Geometry check sheet. Reference: the model listing, model coordinates, mm. A direction names the side the tool comes from. Coordinates: 2 decimals unless noted, no trailing zeros. Write each loop counter-clockwise with the first axis right and the second up, starting at its lowest first coordinate (ties: lowest second). Pieces come first, ordered by that corner, then holes. Notation, with made-up numbers: (39, -12) -> (81, -12) arc R23 ccw to (81, 12) -> close; hole circle Ø4 at (10, 69.25). An arc over 180 degrees is marked (long way). One line per question, with ' | ' between items.
from build123d import *

# Parameters (mm, degrees)
F1_DEPTH = 25


with BuildPart() as f1:
    # F0 (on Right) → F1 (new body)
    with BuildSketch(Plane.YZ):
        with BuildLine():
            ThreePointArc((-42.22845, 60.540393), (-37.159315, 143.848694), (-61.121118, 223.797434))
            Line((-61.121118, 223.797434), (-85.621118, 223.797434))
            Line((-85.621118, 223.797434), (-85.621118, 299.997434))
            Line((-85.621118, 299.997434), (-110.621118, 299.997434))
            Line((-110.621118, 299.997434), (-110.621118, 224.997434))
            ThreePointArc((-110.621118, 224.997434), (-79.816037, 145.650842), (-78.79324, 60.540393))
            ThreePointArc((-78.79324, 60.540393), (-76.894776, -39.398884), (-38.776239, -131.802566))
            Line((-38.776239, -131.802566), (-16.268492, -131.802566))
            ThreePointArc((-16.268492, -131.802566), (-47.291443, -38.066293), (-42.22845, 60.540393))
        make_face()
    extrude(amount=F1_DEPTH)


solid = f1.part
1. Mould release check, pull along Z, two halves, no side actions. Record for faces 3 (the face through (12.325, -47.102, -39.444)), 4 (the face through (12, -28, -131.803)), 5 (the face through (12.325, -77.178, -38.02)), 6 (the face through (25, -67, 85)): released by +Z, released by -Z, zero draft, split by the parting line, or undercut.
Worked answers:
face 3: undercut | face 4: released by -Z | face 5: undercut | face 6: zero draft
2. Cross-section at A-A on x = 17. Record the boundary of the cut face in (y, z).
Worked answers:
outline: (-110.62, 225) arc R238.83 cw to (-78.79, 60.54) arc R270.07 ccw to (-38.78, -131.8) -> (-16.27, -131.8) arc R267.73 cw to (-42.23, 60.54) arc R238.36 ccw to (-61.12, 223.8) -> (-85.62, 223.8) -> (-85.62, 300) -> (-110.62, 300) -> close
3. Material ranges on line 1 (Y direction, x = 7.75, z = 261.5); line 2 (Y direction, x = 1.5, z = 125.5); line 3 (Z direction, x = 9.25, y = -63.5), recorded low to high. Write a range as from..to.
Worked answers:
line 1: -110.62..-85.62 | line 2: -76.8..-35.75 | line 3: -84.04..223.8
4. Cross-section at B-B on z = 267.5. Record the boundary of the cut face in (x, y).
Worked answers:
outline: (0, -110.62) -> (25, -110.62) -> (25, -85.62) -> (0, -85.62) -> close
5. Tool access check on faces 1 (the face through (12, -85.621, 261)), 2 (the face through (12.325, -37.027, 142.682)). Record the directions out of +Z, -Z, +X, -X, +Y, -Y that give a thin tool (end or side, any length) a straight path to the whole face; none if there is none.
Worked answers:
face 1: +Z, +X, -X, +Y | face 2: +X, -X, +Y
6. Cross-section at C-C on y = -57.5. Record the boundary of the cut face in (x, z).
Worked answers:
outline: (0, -97.99) -> (25, -97.99) -> (25, 216.3) -> (0, 216.3) -> close
7. Go/stop test with flat-tipped pins: P1, Ø8, axis at x = 11, y = -75.5, coming from the +Z side; P2, Ø12, axis at x = 13.5, z = 211, coming from the -Y side; P3, Ø12, axis at x = 17, z = -75.5, coming from the +Y side. Record where each tip stops, or that it passes through.
Worked answers:
P1: z = 223.8 | P2: y = -105.93 | P3: y = -37.7
